Source: CAD feature listing. Evaluate the final solid. Frame: model axes, mm. Coordinates: 2 decimals unless noted, no trailing zeros. Order: outer loops, then holes, each group sorted by start corner. A loop starts at its lowest first (then second) coordinate and runs counter-clockwise, first axis right, second up.
Item 1: Section C-C on x = -1. Return the cut outline in (y, z).
Item 2: Section A-A on x = 15.75. Return the cut outline in (y, z).
Item 3: Ray query, line 1 (Y direction, x = -11.5, z = -3.75); line 2 (X direction, y = 2.25, z = -8). Return the intervals inside material, ascending.
Item 4: Section B-B on z = -5.35. Return the cut outline in (x, y).
Item 5: Contact query for a flat-ended pin moving along its axis: P1, Ø9.5, axis at x = -8.5, z = 1.5, coming from the -Y side. Output: stop coordinate, or through.
Item 6: Section D-D on z = -2.75. Return the cut outline in (x, y), then the cut area to 3 significant figures.
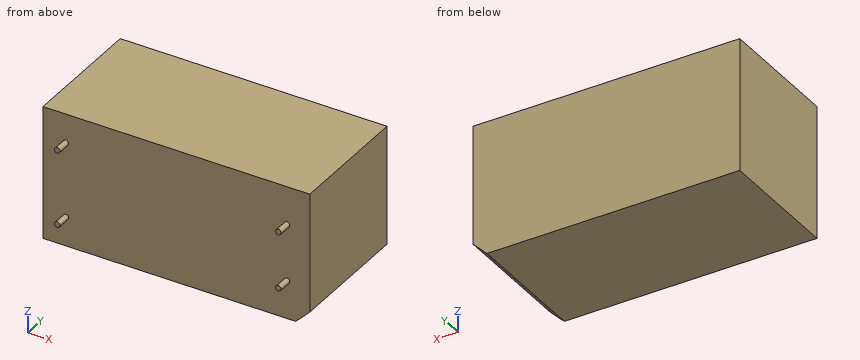
from build123d import *

# Parameters (mm, degrees)
EXTRUDE_1_DEPTH = 18
SKETCH_2_R      = 0.4
EXTRUDE_2_DEPTH = 2


with BuildPart() as part:
    # Эскиз1 → Бобышка-Вытянуть1 (new body)
    with BuildSketch(Plane(origin=(0, 0, 0), x_dir=(1, 0, 0), z_dir=(0, 1, 0))):
        Polygon((19, -9.5), (19, 7.5), (17, 9.5), (-19, 9.5), (-19, -9.5), align=None)
    extrude(amount=EXTRUDE_1_DEPTH)

    # Эскиз2 → Бобышка-Вытянуть2 (add)
    with BuildSketch(Plane.XZ):
        with Locations(Location((-15.75, 5.35, 0), (0, 0, 270))):
            Circle(SKETCH_2_R)
        with Locations(Location((-15.75, -5.35, 0), (0, 0, 270))):
            Circle(SKETCH_2_R)
        with Locations(Location((15.75, 4.05, 0), (0, 0, 270))):
            Circle(SKETCH_2_R)
        with Locations(Location((15.75, -4.05, 0), (0, 0, 270))):
            Circle(SKETCH_2_R)
    extrude(amount=EXTRUDE_2_DEPTH)


solid = part.part
Answer list:
1. outline: (0, -9.5) - (18, -9.5) - (18, 9.5) - (0, 9.5) - close
2. outline: (-2, -4.45) - (0, -4.45) - (0, -9.5) - (18, -9.5) - (18, 9.5) - (0, 9.5) - (0, 4.45) - (-2, 4.45) - (-2, 3.65) - (0, 3.65) - (0, -3.65) - (-2, -3.65) - close
3. line 1: y = 0 to 18
3. line 2: x = -19 to 18.5
4. outline: (-19, 0) - (-16.15, 0) - (-16.15, -2) - (-15.35, -2) - (-15.35, 0) - (19, 0) - (19, 18) - (-19, 18) - close
5. P1: stops at y = 0
6. outline: (-19, 0) - (19, 0) - (19, 18) - (-19, 18) - close
6. area: 684 mm2
